Could you check a few things on this model? Use its own coordinates, in mm. A direction names the side the tool comes from. Coordinates: 2 decimals unless noted, no trailing zeros. Loops run counter-clockwise (first coordinate to the right, second up) from the corner with the lowest first, then second, coordinate; pieces in that order, holes last.
1) Imagine slicing it at D-D on z = 0.25. Please give me the cut outline in (x, y) (3 decimals).
2) Imagine slicing it at C-C on y = -1.4. Please give me the cut outline in (x, z), plus the area to 3 significant figures.
3) Thinking about a two-plate mould opening in Z: for faces 1 (the face through (0, 0, 1)), 2 (the face through (0, 0, -0.5)), 3 (the face through (5.296, -0.086, -0.746)), 4 (the face through (-5.237, -1.445, 0.007)), which applies, released by +Z, released by -Z, zero draft, split by the parting line, or undercut?
4) For faces 5 (the face through (-5.85, 0.09, -0.75)), 6 (the face through (4.99, -0.91, 0.01)), which set-ups out of +Z, -Z, +X, -X, +Y, -Y let a thin tool reach every point of the face, with its end or its side?
5) If I drill on line 1 along X through (y, z) = (-0.05, 0.85); line 2 along X through (y, z) = (-0.3, 0.1); line 3 along X through (y, z) = (-0.6, 0.75), over which ranges is the centre line in solid material (lowest first)?
6) Imagine slicing it at B-B on x = -0.5. Please give me the cut outline in (y, z).
7) Will this pin go through, and if not, where does the flat tip stop? P1, Ø2.5, axis at x = 2.8, y = 0, coming from the -Z side.
8) Imagine slicing it at A-A on y = 0. Please give me the cut outline in (x, z).
Solid Edge part; units mm, degrees
sketch "Sketch1" plane through (0, 0, 0) normal (0, 0, 1) x (1, 0, 0)
  circle A0 centre (-3.3526, 0) radius 2.375
  circle A1 centre (2.7974, 0) radius 2.375
extrude "Protrusion1" add sketch "Sketch1" along normal mid plane 1
sketch "Sketch2" plane through (-3.3526, 0, -0.5) normal (0, 0, -1) x (0, -1, 0)
  arc A0 (-1.5841, -1.9351) -> (-1.5839, -4.2158) centre (-2.5177, -3.0755) cw
  arc A1 (1.5841, -1.9351) -> (1.5839, -4.2158) centre (2.5177, -3.0755) ccw
  arc A2 (1.5841, -1.9351) -> (-1.5841, -1.9351) centre (0, 0) ccw
  arc A3 (-1.5839, -4.2158) -> (1.5839, -4.2158) centre (0, -6.15) ccw
extrude "ExtrudedProtrusion_5" add sketch "Sketch2" along normal blind 0.5
mirror "Mirror1" about plane through (0, 0, 0) normal (0, 0, 1) of "ExtrudedProtrusion_5"
hole "Hole_5" at (-3.3526, 0, 1) direction (0, 0, -1) diameter 2.25 end up to next
hole "Hole1" at (2.7974, 0, 1) direction (0, 0, -1) diameter 2.25 end up to next
Filled in:
1. outline: circle Ø4.75 at (-3.353, 0); circle Ø4.75 at (2.797, 0); hole circle Ø2.25 at (-3.353, 0); hole circle Ø2.25 at (2.797, 0)
2. outline: (-5.42, -1) - (-1.24, -1) - (-1.24, -0.5) - (-1.43, -0.5) - (-1.43, 0.5) - (-1.24, 0.5) - (-1.24, 1) - (-5.42, 1) - (-5.42, 0.5) - (-5.27, 0.5) - (-5.27, -0.5) - (-5.42, -0.5) - close; (0.68, -1) - (4.87, -1) - (4.87, -0.5) - (4.72, -0.5) - (4.72, 0.5) - (4.87, 0.5) - (4.87, 1) - (0.68, 1) - (0.68, 0.5) - (0.88, 0.5) - (0.88, -0.5) - (0.68, -0.5) - close
2. area: 16.0 mm2
3. face 1: released by +Z
3. face 2: undercut
3. face 3: zero draft
3. face 4: undercut
4. face 5: +Z, -Z
4. face 6: none
5. line 1: x = -5.85 to -4.48, -2.23 to 1.67, 3.92 to 5.3
5. line 2: x = -5.71 to -4.44, -2.27 to -1, 0.44 to 1.71, 3.88 to 5.15
5. line 3: x = -5.78 to -4.3, -2.4 to 1.85, 3.75 to 5.22
6. outline: (-1.06, -1) - (1.06, -1) - (1.06, -0.5) - (-1.06, -0.5) - close; (-1.06, 0.5) - (1.06, 0.5) - (1.06, 1) - (-1.06, 1) - close
7. P1: stops at z = -1
8. outline: (-5.85, -1) - (-4.48, -1) - (-4.48, 1) - (-5.85, 1) - (-5.85, 0.5) - (-5.73, 0.5) - (-5.73, -0.5) - (-5.85, -0.5) - close; (-2.23, -1) - (1.67, -1) - (1.67, 1) - (-2.23, 1) - close; (3.92, -1) - (5.3, -1) - (5.3, -0.5) - (5.17, -0.5) - (5.17, 0.5) - (5.3, 0.5) - (5.3, 1) - (3.92, 1) - close; hole (-0.98, -0.5) - (0.42, -0.5) - (0.42, 0.5) - (-0.98, 0.5) - close
